Source: CAD feature listing. Evaluate the final solid. Frame: model axes, mm. Face numbers are marked on the shaded views. A direction names the side the tool comes from. Round coordinates to 2 decimals unless told otherwise and drop trailing zeros. Loops run counter-clockwise (first coordinate to the right, second up) from the corner with the lowest first, then second, coordinate; pieces in that order, holes last. Notation, with made-up numbers: M -10,44 L 3,44 A15 cw 3,48 Z; hole C 47.5,-30 d1. An arc over 180 degrees is marked long. Answer as a JSON object with one key per item and string values.
from build123d import *

# Parameters (mm, degrees)
F1_DEPTH = 20


with BuildPart() as f1:
    # F0 (on Top) → F1 (new body)
    with BuildSketch(Plane.XY):
        Polygon((22.4, 1.568319), (21, 2.068319), (21, -2.068319), (22.4, -1.431681), align=None)
        Polygon((21, -2.068319), (21, 2.068319), (20.192982, 6.125474), (18.609959, 9.94723), (16.311765, 13.38672), (13.38672, 16.311765), (9.94723, 18.609959), (6.125474, 20.192982), (2.068319, 21), (-2.068319, 21), (-6.125474, 20.192982), (-9.94723, 18.609959), (-13.38672, 16.311765), (-16.311765, 13.38672), (-18.609959, 9.94723), (-20.192982, 6.125474), (-21, 2.068319), (-21, -2.068319), (-20.192982, -6.125474), (-18.609959, -9.94723), (-16.311765, -13.38672), (-13.38672, -16.311765), (-9.94723, -18.609959), (-6.125474, -20.192982), (-2.068319, -21), (2.068319, -21), (6.125474, -20.192982), (9.94723, -18.609959), (13.38672, -16.311765), (16.311765, -13.38672), (18.609959, -9.94723), (20.192982, -6.125474), align=None)
        Polygon((18.609959, 9.94723), (20.192982, 6.125474), (21.242782, 7.249409), (20.094732, 10.021047), align=None)
        Polygon((21.295071, -7.123171), (20.192982, -6.125474), (18.609959, -9.94723), (20.147021, -9.894809), align=None)
        Polygon((13.38672, 16.311765), (16.311765, 13.38672), (16.851543, 14.826841), (14.730223, 16.948161), align=None)
        Polygon((16.948161, -14.730223), (16.311765, -13.38672), (13.38672, -16.311765), (14.826841, -16.851543), align=None)
        Polygon((6.125474, 20.192982), (9.94723, 18.609959), (9.894809, 20.147021), (7.123171, 21.295071), align=None)
        Polygon((10.021047, -20.094732), (9.94723, -18.609959), (6.125474, -20.192982), (7.249409, -21.242782), align=None)
        Polygon((-2.068319, 21), (2.068319, 21), (1.431681, 22.4), (-1.568319, 22.4), align=None)
        Polygon((1.568319, -22.4), (2.068319, -21), (-2.068319, -21), (-1.431681, -22.4), align=None)
        Polygon((-9.94723, 18.609959), (-6.125474, 20.192982), (-7.249408, 21.242782), (-10.021047, 20.094732), align=None)
        Polygon((-7.123171, -21.295071), (-6.125474, -20.192982), (-9.94723, -18.609959), (-9.894809, -20.147021), align=None)
        Polygon((-16.311765, 13.38672), (-13.38672, 16.311765), (-14.826841, 16.851543), (-16.948161, 14.730223), align=None)
        Polygon((-14.730223, -16.948161), (-13.38672, -16.311765), (-16.311765, -13.38672), (-16.851543, -14.826841), align=None)
        Polygon((-20.192982, 6.125474), (-18.609959, 9.94723), (-20.147021, 9.894809), (-21.295071, 7.123171), align=None)
        Polygon((-20.094732, -10.021047), (-18.609959, -9.94723), (-20.192982, -6.125474), (-21.242782, -7.249408), align=None)
        Polygon((-21, -2.068319), (-21, 2.068319), (-22.4, 1.431681), (-22.4, -1.568319), align=None)
    extrude(amount=F1_DEPTH)


solid = f1.part
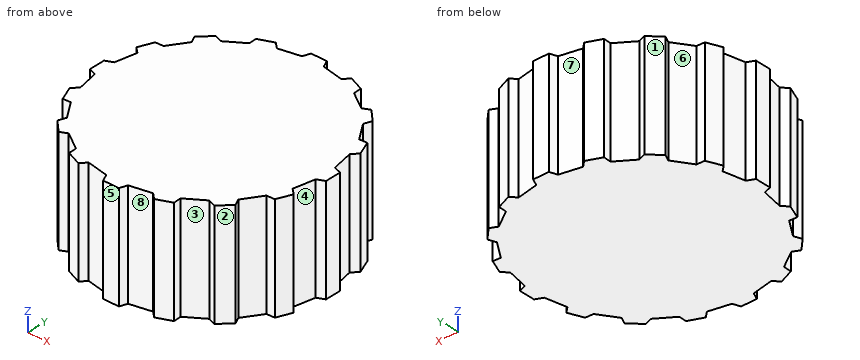
Item 1: Section B-B on y = -5.5. Return the cut outline in (x, z), then the cut area to 3 significant figures.
Answer sheet:
{"outline": "M -20.32,0 L 20.32,0 L 20.32,20 L -20.32,20 Z", "area": "813 mm²"}
Item 2: Section A-A on x = -4.5. Return the cut outline in (y, z), then the cut area to 3 significant figures.
Answer sheet:
{"outline": "M -20.52,0 L 20.52,0 L 20.52,20 L -20.52,20 Z", "area": "821 mm²"}
Item 3: Pull-direction query (X, two-part tool) for the marked faces 1, 2 and 3; classes: pulls with the +X half, pulls with the -X half, needs draft (parallel to the pull), parting line crosses it, or undercut.
Answer sheet:
{"face 1": "pulls with the -X half", "face 2": "pulls with the +X half", "face 3": "undercut"}
Item 4: Access query for the marked faces 4, 5, 6, 7 and 8. Directions: +Z, -Z, +X, -X, +Y, -Y. A direction counts if a zero-diameter tool reaches every point of the face in a straight line with its end or side. Return the directions, or none.
Answer sheet:
{"face 4": "+Z, -Z, +X", "face 5": "+Z, -Z, +X, -X, -Y", "face 6": "+Z, -Z, -X", "face 7": "+Z, -Z, +Y", "face 8": "+Z, -Z, -Y"}
Item 5: Contact query for flat-ended pins moving along their axis: pin 1 Ø2 at (x, z) = (-8.5, 8) entering from +Y; pin 2 Ø6 at (x, y) = (-8, 2) entering from -Z; pin 3 Ø1.5 at (x, z) = (-16, 11) entering from -Y; pin 4 Ø6 at (x, z) = (17.5, 4.5) entering from +Y. Output: stop coordinate, or through.
Answer sheet:
{"pin 1": "stops at y = 21.14", "pin 2": "stops at z = 0", "pin 3": "stops at y = -16.43", "pin 4": "stops at y = 16.95"}
Item 6: Line query: probe 1 along X at (y, z) = (-6, 10.5); probe 2 along Y at (x, z) = (7.5, 16.5); probe 3 along X at (y, z) = (-11, 17). Output: solid intervals per line, ascending. Write a range as from..to.
Answer sheet:
{"probe 1": "x = -20.22..20.22", "probe 2": "y = -21.14..21.14", "probe 3": "x = -17.91..17.91"}
